Input: part model. Units: mm. Frame: model coordinates. Coordinates: 2 decimals unless noted, no trailing zeros. Write each loop counter-clockwise with the first axis right and the second up, starting at its lowest first coordinate (ties: lowest second). Pieces come first, ordered by that corner, then holes. Notation, with made-up numbers: (-1.75, -20.5) - (51.25, -20.5) arc R23 ccw to (51.25, 4.5) - close; hole circle Ø1 at (26, -20). An arc over 180 degrees is marked (long way). Put each result on its own line as item: value. Start each with the question number.
1. Cut plane A-A, the plane x = 71. Return loops of the section in (y, z).
2. Line query: line 1 (X direction, y = -42, z = -18.5); line 2 (Z direction, x = -69.5, y = -51.5); line 3 (X direction, y = -66.5, z = -18). Output: solid intervals per line, ascending.
3. Pin query (flat end, axial travel): pin 1 (6 mm diameter, centred on y = -38.5, z = -9, fed in from +X); pin 2 (2 mm diameter, centred on y = -50, z = 0.5, fed in from -X); pin 3 (4 mm diameter, centred on y = -59, z = -8.5, fed in from -X). Return the tip coordinate at first contact, or that it passes through.
4. Cut plane B-B, the plane x = 40.5. Return loops of the section in (y, z).
from build123d import *

# Parameters (mm, degrees)
F1_DEPTH = 100
F3_DEPTH = 100.0010001


with BuildPart() as f1:
    # F0 (on Front) → F1 (new body)
    with BuildSketch(Plane.XZ):
        with BuildLine():
            add(Edge.make_bspline(
                [(-62.5, -20), (-73.1268525124, -20), (-80.4059031562, -7.7978468302), (-84.9233715293, 1.839947371), (-86.2586413814, 7.0207393153)],
                knots=[0, 0, 0, 0, 0.5386149438, 1, 1, 1, 1], degree=3))
            Line((-62.5, -20), (81.9273708606, -20))
            ThreePointArc((81.9273708606, -20), (85.2753510448, -18.1888418596), (85.5914704468, -14.3955143432))
            add(Edge.make_bspline(
                [(85.5914704468, -14.3955143432), (80.4923521492, -2.7508622611), (61.7807143057, 13.6061614536), (50.4547609094, 18.5615463365), (-2.3409408703, 16.1806235265), (-42.1157825532, 18.1611356538), (-69.9472957559, 14.7146056584), (-84.4380939102, 11.0206353633)],
                knots=[0.0286493497, 0.0286493497, 0.0286493497, 0.0286493497, 0.2113092276, 0.3338194515, 0.5678984107, 0.7846695753, 1, 1, 1, 1], degree=3))
            ThreePointArc((-84.4380939102, 11.0206353633), (-86.219889206, 9.4173592411), (-86.2586413814, 7.0207393153))
        make_face()
    extrude(amount=F1_DEPTH)

    # F2 (on face) → F3 (cut, through all)
    with BuildSketch(Plane.XZ.offset(100)):
        with BuildLine():
            Line((76.7807810103, -12.2087626863), (81.9273708606, -20))
            Line((81.9273708606, -20), (89.4811376929, -23.3435314149))
            Line((89.4811376929, -23.3435314149), (91.3648977876, -5.6361360475))
            Line((91.3648977876, -5.6361360475), (72.1504986286, 22.6203482598))
            Line((72.1504986286, 22.6203482598), (18.2747989893, 25.8227474988))
            Line((18.2747989893, 25.8227474988), (-74.9715939164, 17.3458047211))
            Line((-74.9715939164, 17.3458047211), (-69.5344796887, 14.1921793268))
            Line((-69.5344796887, 14.1921793268), (34.6666465938, 14.1921793268))
            ThreePointArc((34.6666465938, 14.1921793268), (58.5861493226, 5.5577951747), (76.7807810103, -12.2087626863))
        make_face()
    extrude(amount=-F3_DEPTH, mode=Mode.SUBTRACT)


solid = f1.part
Report:
1. outline: (-100, -20) - (0, -20) - (0, -4.79) - (-100, -4.79) - close
2. line 1: x = -70.24 to 80.94
2. line 2: z = -18.81 to 14.19
2. line 3: x = -71.26 to 80.61
3. pin 1: stops at x = 76.64
3. pin 2: stops at x = -84.47
3. pin 3: stops at x = -80.75
4. outline: (-100, -20) - (0, -20) - (0, 13.12) - (-100, 13.12) - close
